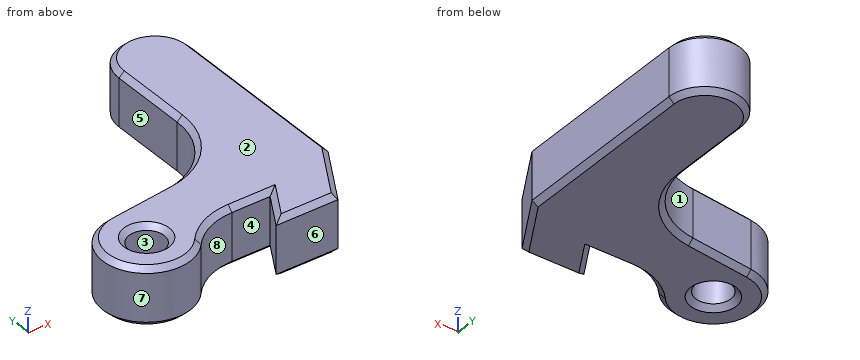
from build123d import *

# Parameters (mm, degrees)
CROQUIS1_R              = 1.7
SALIENTE_EXTRUIR4_DEPTH = 5.6
CHAFL_N3_SIZE           = 0.5


with BuildPart() as part:
    # Croquis1 → Saliente-Extruir4 (new body)
    with BuildSketch(Plane.XY):
        with BuildLine():
            Line((16.09779672, 23.748075599), (16.09779672, 16.177387183))
            ThreePointArc((16.09779672, 16.177387183), (14.340486657, 11.539046724), (9.9508818, 9.229564082))
            Line((9.9508818, 9.229564082), (3.735387364, 8.46639762))
            ThreePointArc((3.735387364, 8.46639762), (0.50668224, 2.230828662), (7.490439371, 1.500080182))
            ThreePointArc((7.490439371, 1.500080182), (9.545533222, 3.0653793), (12.068287742, 3.621510305))
            Line((12.068287742, 3.621510305), (15.766559407, 3.621510305))
            Line((15.766559407, 3.621510305), (13.745833465, 0.121510305))
            Line((13.745833465, 0.121510305), (19.750276265, 0.121510305))
            Line((19.750276265, 0.121510305), (23.097796776, 5.919585909))
            Line((23.097796776, 5.919585909), (23.097796776, 23.748075599))
            ThreePointArc((23.097796776, 23.748075599), (19.597796748, 27.248075627), (16.09779672, 23.748075599))
        make_face()
        with Locations((4.247796776, 4.247400512)):
            Circle(CROQUIS1_R, mode=Mode.SUBTRACT)
    extrude(amount=SALIENTE_EXTRUIR4_DEPTH)

    # Chaflán3
    chafl_n3_edges = [part.edges().sort_by_distance(p)[0] for p in [
        (14.340486657, 11.539046724, 5.6),
        (23.097796776, 14.833830754, 0),
        (21.42403652, 3.020548107, 0),
        (16.748054865, 0.121510305, 0),
        (14.756196436, 1.871510305, 0),
        (13.917423575, 3.621510305, 0),
        (9.545533222, 3.0653793, 0),
        (0.50668224, 2.230828662, 0),
        (6.843134582, 8.847980851, 0),
        (6.843134582, 8.847980851, 5.6),
        (14.340486657, 11.539046724, 0),
        (16.09779672, 19.962731391, 0),
        (19.597796748, 27.248075627, 0),
        (0.50668224, 2.230828662, 5.6),
        (9.545533222, 3.0653793, 5.6),
        (13.917423575, 3.621510305, 5.6),
        (14.756196436, 1.871510305, 5.6),
        (2.547796776, 4.247400512, 0),
        (2.547796776, 4.247400512, 5.6),
        (16.748054865, 0.121510305, 5.6),
        (21.42403652, 3.020548107, 5.6),
        (23.097796776, 14.833830754, 5.6),
        (19.597796748, 27.248075627, 5.6),
        (16.09779672, 19.962731391, 5.6),
    ]]
    chamfer(chafl_n3_edges, length=CHAFL_N3_SIZE)


solid = part.part
Here's how the part is built. I have some questions about the finished solid (model axes, mm). Face numbers are marked on the shaded views. A direction names the side the tool comes from. Round coordinates to 2 decimals unless told otherwise and drop trailing zeros. Loops run counter-clockwise (first coordinate to the right, second up) from the corner with the lowest first, then second, coordinate; pieces in that order, holes last.
1. If we section it at B-B on y = 22.25: Write out the boundary of the cut face in (x, z).
Answer list:
outline: (16.1, 0.5) - (16.6, 0) - (22.6, 0) - (23.1, 0.5) - (23.1, 5.1) - (22.6, 5.6) - (16.6, 5.6) - (16.1, 5.1) - close
2. For P1, Ø3, axis at x = 14.5, z = 3, coming from the -Y side; P2, Ø2, axis at x = 4.25, y = 4.25, coming from the -Z side, each with a flat end and sliding along its axis, tell me the tip position at first contact or that it passes through.
Answer list:
P1: stops at y = 0.12
P2: passes through
3. Which directions (+Z, -Z, +X, -X, +Y, -Y) give clear straight access to the entire face, cutting with the end or side of a thin tool? Please do the marked faces 5, 6, 7 and 8.
Answer list:
face 5: +Z, -Z, -X, +Y
face 6: +Z, -Z, +X, -Y
face 7: +Z, -Z
face 8: +Z, -Z, -Y
4. If we section it at A-A on z = 4.45: Write out the boundary of the cut face in (x, y), plus the area to 3 significant figures.
Answer list:
outline: (3.74, 8.47) arc R4.25 ccw (long way) to (7.49, 1.5) arc R6 cw to (12.07, 3.62) - (15.77, 3.62) - (13.75, 0.12) - (19.75, 0.12) - (23.1, 5.92) - (23.1, 23.75) arc R3.5 ccw to (16.1, 23.75) - (16.1, 16.18) arc R7 cw to (9.95, 9.23) - close; hole circle Ø3.4 at (4.25, 4.25)
area: 287 mm2
5. If I drill on line 1 along X through (y, z) = (21.5, 0.95); line 2 along X through (y, z) = (4.75, 4.8); line 3 along X through (y, z) = (1.5, 5), over which ranges is the centre line in solid material (lowest first)?
Answer list:
line 1: x = 16.1 to 23.1
line 2: x = 0.03 to 2.62, 5.87 to 22.42
line 3: x = 1.01 to 7.49, 14.54 to 20.55
6. We'd pull the mould along X, two halves only. Please class the marked faces 1, 2, 3 and 4: +X half, -X half, draft (parallel to the pull), parting line (faces both ways), or undercut.
Answer list:
face 1: -X half
face 2: draft
face 3: undercut
face 4: undercut
